CAD build for the part. Positions are in the model's coordinates, mm. A direction names the side the tool comes from. Give positions to 0.01 mm unless a question says otherwise; leave off trailing zeros. Loops run counter-clockwise (first coordinate to the right, second up) from the corner with the lowest first, then second, coordinate; pieces in that order, holes last. Notation, with made-up numbers: (-38, -30.75) -> (17, -30.75) arc R12 cw to (17, -24.75) -> close; hole circle Ø3 at (66.25, 86.25). An arc over 180 degrees is marked (long way). Use one line per item in the form item = value.
```python
from build123d import *

# Parameters (mm, degrees)
SKETCH_1_W         = 7
SKETCH_1_H         = 20
EXTRUDE_1_DEPTH    = 140
SKETCH_2_W         = 15
SKETCH_2_H         = 12
EXTRUDE_2_DEPTH    = 10
HOLE_WIZARD_M4_1_D = 3.3


with BuildPart() as part:
    # 草图1 → 凸台-拉伸1 (new, symmetric)
    with BuildSketch(Plane(origin=(0, 0, 0), x_dir=(0, 0, -1), z_dir=(1, 0, 0))):
        Rectangle(SKETCH_1_W, SKETCH_1_H)
    extrude(amount=EXTRUDE_1_DEPTH, both=True)

    # 草图2 → 凸台-拉伸2 (add)
    with BuildSketch(Plane.XY.offset(3.5)):
        with Locations((-117.5, 4)):
            Rectangle(SKETCH_2_W, SKETCH_2_H)
    extrude_2 = extrude(amount=EXTRUDE_2_DEPTH)

    # 镜向1: 凸台-拉伸2 across plane
    add(extrude_2.mirror(Plane(origin=(0, 0, 0), x_dir=(0, 0, 1), z_dir=(1, 0, 0))))

    # M4 螺纹孔1 (through all)
    with Locations(Plane(origin=(0, -2, 0), x_dir=(-1, 0, 0), z_dir=(0, -1, 0))):
        with Locations((-117.5, -8.5), (117.5, -8.5)):
            Hole(HOLE_WIZARD_M4_1_D / 2)


solid = part.part
```
1. Tool access for faces 5 (the flat face through (-119.3, -2, 8.4)), 6 (the flat face through (-110, 4, 8)), 7 (the flat face through (118, 4, 13.5)): list every direction of +Z, -Z, +X, -X, +Y, -Y with a clear straight run to the whole face (end or side of a thin tool).
Result sheet:
face_5 = +Z, +X, -X, -Y
face_6 = +Z, +Y, -Y
face_7 = +Z, +X, -X, +Y, -Y
2. Drill centre lines: line 1 (X direction, y = 2, z = 8.5); line 2 (Z direction, x = 117.5, y = 6); line 3 (X direction, y = 2.75, z = 12). Where is each one in solid material? Low to high.
Result sheet:
line_1 = -125 to -119.15, -115.85 to -110, 110 to 115.85, 119.15 to 125
line_2 = -3.5 to 6.85, 10.15 to 13.5
line_3 = -125 to -110, 110 to 125
3. Cut at B-B, the plane x = -62.5. Write the cut outline in (y, z), then the cut area to 3 significant figures.
Result sheet:
outline = (-10, -3.5) -> (10, -3.5) -> (10, 3.5) -> (-10, 3.5) -> close
area = 140 mm^2
4. Cut at A-A, the plane y = 7.25. Write the cut outline in (x, z).
Result sheet:
outline = (-140, -3.5) -> (140, -3.5) -> (140, 3.5) -> (125, 3.5) -> (125, 13.5) -> (110, 13.5) -> (110, 3.5) -> (-110, 3.5) -> (-110, 13.5) -> (-125, 13.5) -> (-125, 3.5) -> (-140, 3.5) -> close; hole circle Ø3.3 at (-117.5, 8.5); hole circle Ø3.3 at (117.5, 8.5)
5. Cut at C-C, the plane y = -6. Write the cut outline in (x, z), then the cut area to 3 significant figures.
Result sheet:
outline = (-140, -3.5) -> (140, -3.5) -> (140, 3.5) -> (-140, 3.5) -> close
area = 1,960 mm^2
6. Drop flat-ended pins along their axis: P1, Ø5, axis at x = 26.5, y = 2.5, coming from the +Z side; P2, Ø3, axis at y = 3.5, z = 7.5, coming from the -X side; P3, Ø4.5, axis at x = 117.5, z = 8.5, coming from the -Y side. Give the stop position or say it passes through.
Result sheet:
P1 = 3.5
P2 = -125
P3 = -2
7. Mould opens along X. For faces 1 (the flat face through (-125, 4, 8)), 2 (the flat face through (2, -10, 0)), 3 (the flat face through (110, 4, 8)), 4 (the flat face through (125, 4, 8)) say: pulls with the +X half, pulls with the -X half, needs draft (parallel to the pull), parting line crosses it, or undercut.
Result sheet:
face_1 = pulls with the -X half
face_2 = needs draft
face_3 = undercut
face_4 = pulls with the +X half
